CAD build for the part. Positions are in the model's coordinates, mm. Face numbers are marked on the shaded views. A direction names the side the tool comes from. Round coordinates to 2 decimals unless told otherwise and drop trailing zeros. Order: outer loops, then holes, each group sorted by start corner. A loop starts at its lowest first (then second) coordinate and runs counter-clockwise, first axis right, second up. Notation, with made-up numbers: M 52.5,25 L 82.5,25 A20 cw 82.5,32 Z; hole C -14.5,21 d6. An arc over 180 degrees is marked long. Answer as CSV lines item,"result". Start each with the question number.
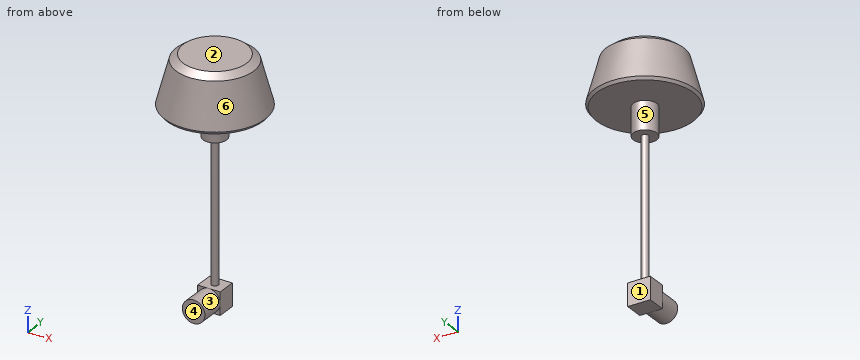
```python
from build123d import *

# Parameters (mm, degrees)
F0_R     = 4
F1_DEPTH = 4.25
F2_W     = 8
F2_H     = 8
F3_DEPTH = 6.7
F4_R     = 1.25
F5_DEPTH = 50
F6_R     = 4.15
F7_DEPTH = 10
F8_R     = 18
F8_R_2   = 4.15
F9_DEPTH = 18
F9_TAPER = 15


# Not quite as in the source:
# - a fillet or chamfer that OpenCascade refuses, or shapes differently, is made with other operations: its cross-section is extruded or revolved along the edge and cut away or added


with BuildPart() as f1:
    # F0 (on Front) → F1 (new body, symmetric)
    with BuildSketch(Plane.XZ):
        Circle(F0_R)
    extrude(amount=F1_DEPTH, both=True)

    # F2 (on face) → F3 (join)
    with BuildSketch(Plane(origin=(0, 4.25, 0), x_dir=(-1, 0, 0), z_dir=(0, 1, 0))):
        Rectangle(F2_W, F2_H)
    extrude(amount=F3_DEPTH)

    # F4 (on face) → F5 (join)
    with BuildSketch(Plane.XY.offset(4)):
        with Locations((0, 7.6)):
            Circle(F4_R)
    extrude(amount=F5_DEPTH)

    # F6 (on face) → F7 (join)
    with BuildSketch(Plane.XY.offset(54)):
        with Locations((0, 7.6)):
            Circle(F6_R)
    extrude(amount=F7_DEPTH)

    # F8 (on face) → F9 (join)
    with BuildSketch(Plane.XY.offset(64)):
        with Locations((0, 7.6)):
            Circle(F8_R)
        with Locations((0, 7.6)):
            Circle(F8_R_2, mode=Mode.SUBTRACT)
        with Locations((0, 7.6)):
            Circle(F8_R_2)
    extrude(amount=F9_DEPTH, taper=F9_TAPER)

    # F10: chamfer of 1 on 1 edges, made by hand

    # F10_s1 → F10_t2 (revolve, cut)
    with BuildSketch(Plane.XZ.offset(-7.6)):
        Polygon((17, 64), (17.7411809549, 64.9659258263), (18, 64), align=None)
    revolve(axis=Axis((0, 7.6, 64), (0, 0, -1)), mode=Mode.SUBTRACT)

    # F11: chamfer of 2 on 1 edges, made by hand

    # F11_s1 → F11_t2 (revolve, cut)
    with BuildSketch(Plane.XZ.offset(-7.6)):
        Polygon((13.6945526264, 80.0681483474), (11.1769145362, 82), (13.1769145362, 82), align=None)
    revolve(axis=Axis((0, 7.6, 82), (0, 0, -1)), mode=Mode.SUBTRACT)


solid = f1.part
```
Q1. Mould opens along Z. For the marked faces 1, 2 and 3 say: +Z half, -Z half, draft (parallel to the pull), parting line (faces both ways), or undercut.
Q2. Band-saw the part on C-C, the plane z = 18.5. Write the cut outline in (x, y).
Q3. Probe line 1 along Z through (x, y) = (2.5, 5.5); line 2 along Y through (x, z) = (-1.5, 3); line 3 along Z through (x, y) = (7.5, 0.5). List the from-to ranges inside material, lowest first. Write a range as from..to.
Q4. Band-saw the part on B-B, the plane z = 1. Write the cut outline in (x, y), then the cut area to 3 significant figures.
Q5. Band-saw the part on A-A, the plane y = 7.6. Write the cut outline in (x, z).
Q6. Drop flat-ended pins along their axis: P1, Ø3.5, axis at y = 6.5, z = -1.5, coming from the +X side; P2, Ø4.5, axis at x = -2, z = -2.5, coming from the -Y side; P3, Ø2, axis at x = -6.5, z = 64, coming from the -Y side. Give the stop position or say it passes through.
Q7. Tool access for the marked faces 4, 5 and 6: list every direction of +Z, -Z, +X, -X, +Y, -Y with a clear straight run to the whole face (end or side of a thin tool).
Answer:
1,face 1,"draft"
1,face 2,"+Z half"
1,face 3,"undercut"
2,outline,"C 0,7.6 d2.5"
3,line 1,"z = -4..4, 54..82"
3,line 2,"y = -4.25..10.95"
3,line 3,"z = 64..82"
4,outline,"M -4,4.25 L -3.87,4.25 L -3.87,-4.25 L 3.87,-4.25 L 3.87,4.25 L 4,4.25 L 4,10.95 L -4,10.95 Z"
4,area,"119 mm^2"
5,outline,"M -17.74,64.97 L -17,64 L -4.15,64 L -4.15,54 L -1.25,54 L -1.25,4 L -4,4 L -4,-4 L 4,-4 L 4,4 L 1.25,4 L 1.25,54 L 4.15,54 L 4.15,64 L 17,64 L 17.74,64.97 L 13.69,80.07 L 11.18,82 L -11.18,82 L -13.69,80.07 Z"
6,P1,"stops at x = 4"
6,P2,"stops at y = -4.25"
6,P3,"stops at y = -9.02"
7,face 4,"-Z, +X, -X, -Y"
7,face 5,"none"
7,face 6,"+Z"
